```python
from build123d import *

# Parameters (mm, degrees)
CUT_EXTRUDE1_DEPTH      = 19
CUT_EXTRUDE1_DEPTH_BACK = 19
SKETCH2_R               = 3.25
FILLET1_R               = 0.5


with BuildPart() as part:
    # Sketch1 → Revolve1 (revolve)
    with BuildSketch(Plane.XY, mode=Mode.PRIVATE) as revolve1_sk:
        Polygon((-14, 0), (11.3, 0), (11.3, 5), (-4.65, 5), (-4.65, 8), (-14, 8), align=None)
    revolve(revolve1_sk.sketch.rotate(Axis((-1.174323487, 0, 0), (1, 0, 0)), 90), axis=Axis((-1.174323487, 0, 0), (1, 0, 0)))

    # Sketch2 → Cut-Extrude1 (cut, two sides: drawn at the far end of the back side and taken through both)
    with BuildSketch(Plane(origin=(0, 0, 0), x_dir=(0, 0, -1), z_dir=(1, 0, 0)).offset(-CUT_EXTRUDE1_DEPTH_BACK)):
        Circle(SKETCH2_R)
    extrude(amount=CUT_EXTRUDE1_DEPTH + CUT_EXTRUDE1_DEPTH_BACK, mode=Mode.SUBTRACT)

    # Fillet1
    fillet1_edges = [part.edges().sort_by_distance(p)[0] for p in [
        (-14, 0, 3.25),
        (11.3, 0, 3.25),
        (-14, 0, -8),
        (-4.65, 0, -8),
        (11.3, 0, -5),
    ]]
    fillet(fillet1_edges, radius=FILLET1_R)


solid = part.part
```
Work out the finished part from the listing and answer in its coordinate system (mm). A direction names the side the tool comes from. Give positions to 0.01 mm unless a question says otherwise; leave off trailing zeros. Write each loop counter-clockwise with the first axis right and the second up, starting at its lowest first coordinate (ties: lowest second). Pieces come first, ordered by that corner, then holes. Notation, with made-up numbers: (-2, -5.75) - (52, -5.75) arc R35 ccw to (52, 32.25) - close; hole circle Ø7 at (-24.5, -15.75). An arc over 180 degrees is marked (long way). Use one line per item in the form item = value.
1. For faces 1 (the face through (-4.65, 5, -2)), 2 (the face through (-14, 3, 3)), determine the directions among +Z, -Z, +X, -X, +Y, -Y from which every point of the face is accessible in a straight line to the end or side of a thin tool.
Filled in:
face_1 = +X
face_2 = +Z, -Z, -X, +Y, -Y
2. A cutting plane is placed at C-C (x = 2). Write down the section's boundary in (y, z).
Filled in:
outline = circle Ø10 at (0, 0); hole circle Ø6.5 at (0, 0)
3. A cutting plane is placed at A-A (z = 0). Write down the section's boundary in (x, y).
Filled in:
outline = (-14, -7.5) arc R0.5 ccw to (-13.5, -8) - (-5.15, -8) arc R0.5 ccw to (-4.65, -7.5) - (-4.65, -5) - (10.8, -5) arc R0.5 ccw to (11.3, -4.5) - (11.3, -3.75) arc R0.5 ccw to (10.8, -3.25) - (-13.5, -3.25) arc R0.5 ccw to (-14, -3.75) - close; (-14, 3.75) arc R0.5 ccw to (-13.5, 3.25) - (10.8, 3.25) arc R0.5 ccw to (11.3, 3.75) - (11.3, 4.5) arc R0.5 ccw to (10.8, 5) - (-4.65, 5) - (-4.65, 7.5) arc R0.5 ccw to (-5.15, 8) - (-13.5, 8) arc R0.5 ccw to (-14, 7.5) - close
4. Each of these flat-tipped pins is pushed along its axis until it touches: pin 1 Ø8 at (x, z) = (-5.5, -4) entering from -Y; pin 2 Ø1 at (x, z) = (2, -1) entering from +Y; pin 3 Ø1.5 at (x, y) = (-3.5, -5) entering from -Z; pin 4 Ø3 at (x, y) = (-5.5, 4) entering from -Z. Where does it stop, or does it pass through?
Filled in:
pin_1 = -8
pin_2 = 4.97
pin_3 = -2.63
pin_4 = -7.6
5. Determine the mould class of faces 3 (the face through (3, 0, -5)), 4 (the face through (11.3, -4, 1)), 5 (the face through (-1.52, -1.978, 2.579)) for opening direction Y: released by +Y, released by -Y, zero draft, split by the parting line, or undercut.
Filled in:
face_3 = split by the parting line
face_4 = zero draft
face_5 = undercut
6. Consider L1, parallel to Y at x = 4, z = 0; L2, parallel to X at y = -2, z = 6.75; L3, parallel to Z at x = 1, y = -3. Determine where each line is inside the solid, lowest interval first.
Filled in:
L1 = -5 to -3.25, 3.25 to 5
L2 = -14 to -4.65
L3 = -4 to -1.25, 1.25 to 4
